```python
from build123d import *

# Parameters (mm, degrees)
F0_W     = 15
F0_H     = 5.5
F0_R     = 2
F0_W_2   = 5.5
F0_H_2   = 15
F0_W_3   = 55
F0_H_3   = 103
F1_DEPTH = 4
F2_R     = 2.5
F3_R     = 5


# Not quite as in the source:
# - a feature names something its author has since deleted; it is built from what else it names


with BuildPart() as f1:
    # F0 (on Top) → F1 (new body)
    with BuildSketch(Plane.XY):
        Polygon((57.5, 63.25), (32.5, 63.25), (-32.5, 63.25), (-32.5, -63.25), (-32.5, -88.25), (57.5, -88.25), align=None)
        with Locations((-12.5, -78.25)):
            Rectangle(F0_W, F0_H, mode=Mode.SUBTRACT)
        with Locations((-26, -56.25)):
            Circle(F0_R, mode=Mode.SUBTRACT)
        with Locations((-0.25, -56.25)):
            Circle(F0_R, mode=Mode.SUBTRACT)
        with Locations((25.5, -56.25)):
            Circle(F0_R, mode=Mode.SUBTRACT)
        with Locations((47.5, -68.25)):
            Rectangle(F0_W_2, F0_H_2, mode=Mode.SUBTRACT)
        Rectangle(F0_W_3, F0_H_3, mode=Mode.SUBTRACT)
        with Locations((-26, 56.75)):
            Circle(F0_R, mode=Mode.SUBTRACT)
        with Locations((-0.25, 56.75)):
            Circle(F0_R, mode=Mode.SUBTRACT)
        with Locations((47.5, -12.5)):
            Rectangle(F0_W_2, F0_H_2, mode=Mode.SUBTRACT)
        with Locations((25.5, 56.75)):
            Circle(F0_R, mode=Mode.SUBTRACT)
        with Locations((47.5, 43.25)):
            Rectangle(F0_W_2, F0_H_2, mode=Mode.SUBTRACT)
    extrude(amount=F1_DEPTH)

    # F2
    f2_edges = [f1.edges().sort_by_distance(p)[0] for p in [
        (-20, -81, 2),
        (-20, -75.5, 2),
        (-5, -75.5, 2),
        (-5, -81, 2),
        (50.25, -60.75, 2),
        (50.25, -75.75, 2),
        (44.75, -75.75, 2),
        (44.75, -60.75, 2),
        (44.75, -5, 2),
        (50.25, -5, 2),
        (50.25, -20, 2),
        (44.75, -20, 2),
        (44.75, 35.75, 2),
        (44.75, 50.75, 2),
        (50.25, 50.75, 2),
        (50.25, 35.75, 2),
    ]]
    fillet(f2_edges, radius=F2_R)

    # F3
    f3_edges = [f1.edges().sort_by_distance(p)[0] for p in [
        (-32.5, 63.25, 2),
        (-32.5, -88.25, 2),
        (57.5, -88.25, 2),
        (57.5, 63.25, 2),
    ]]
    fillet(f3_edges, radius=F3_R)


solid = f1.part
```
Geometry check sheet. Reference: the model listing, model coordinates, mm. A direction names the side the tool comes from. Give positions to 0.01 mm unless a question says otherwise; leave off trailing zeros. Order: outer loops, then holes, each group sorted by start corner. A loop starts at its lowest first (then second) coordinate and runs counter-clockwise, first axis right, second up. Notation, with made-up numbers: (-1.75, 27.5) - (45.25, 27.5) arc R22 cw to (45.25, 63.5) - close; hole circle Ø1 at (3, 18.5). An arc over 180 degrees is marked (long way). Answer in a Markdown table with one row per item. Add a question column.
Q1. Cross-section at C-C, the plane y = 43.5. Enter the section's corners in (x, z).
Q2. Cross-section at A-A, the plane y = 12. Enter the section's corners in (x, z).
Q3. Cross-section at D-D, the plane x = 25.5. Enter the section's corners in (y, z), then the cut area to 3 significant figures.
Q4. Tool access check on faces 4 (the flat face through (44.75, -68, 2)), 5 (the flat face through (57.5, -13, 2)). Record the directions out of +Z, -Z, +X, -X, +Y, -Y that give a thin tool (end or side, any length) a straight path to the whole face; none if there is none.
Q5. Material ranges on probe 1 along Y at (x, z) = (25.5, 1.3); probe 2 along Y at (x, z) = (47, 0.8); probe 3 along X at (y, z) = (-39.5, 3.85), recorded low to high. Write a range as from..to.
Q6. Gauge pin test, flat end, axial feed: pin 1 (2.5 mm diameter, centred on x = 25.5, y = 56.75, fed in from -Z). Record the tip position at first contact, or that the pin passes through.
Q7. Cross-section at B-B, the plane x = -11.5. Enter the section's corners in (y, z).
Q8. Mould release check, pull along Y, two halves, no side actions. Record for faces 1 (the flat face through (44.75, 43, 2)), 2 (the flat face through (32, -11, 4)), 3 (the cylindrical face through (56, 61.82, 2.03)): pulls with the +Y half, pulls with the -Y half, needs draft (parallel to the pull), parting line crosses it, or undercut.
Check values:
| question | item | result |
|---|---|---|
| 1 | outline | (-32.5, 0) - (-27.5, 0) - (-27.5, 4) - (-32.5, 4) - close; (27.5, 0) - (44.75, 0) - (44.75, 4) - (27.5, 4) - close; (50.25, 0) - (57.5, 0) - (57.5, 4) - (50.25, 4) - close |
| 2 | outline | (-32.5, 0) - (-27.5, 0) - (-27.5, 4) - (-32.5, 4) - close; (27.5, 0) - (57.5, 0) - (57.5, 4) - (27.5, 4) - close |
| 3 | outline | (-88.25, 0) - (-58.25, 0) - (-58.25, 4) - (-88.25, 4) - close; (-54.25, 0) - (-51.5, 0) - (-51.5, 4) - (-54.25, 4) - close; (51.5, 0) - (54.75, 0) - (54.75, 4) - (51.5, 4) - close; (58.75, 0) - (63.25, 0) - (63.25, 4) - (58.75, 4) - close |
| 3 | area | 162 mm^2 |
| 4 | face 4 | +Z, -Z |
| 4 | face 5 | +Z, -Z, +X, +Y, -Y |
| 5 | probe 1 | y = -88.25..-58.25, -54.25..-51.5, 51.5..54.75, 58.75..63.25 |
| 5 | probe 2 | y = -88.25..-75.74, -60.76..-19.99, -5.01..35.76, 50.74..63.25 |
| 5 | probe 3 | x = -32.5..-27.5, 27.5..57.5 |
| 6 | pin 1 | passes through |
| 7 | outline | (-88.25, 0) - (-81, 0) - (-81, 4) - (-88.25, 4) - close; (-75.5, 0) - (-51.5, 0) - (-51.5, 4) - (-75.5, 4) - close; (51.5, 0) - (63.25, 0) - (63.25, 4) - (51.5, 4) - close |
| 8 | face 1 | undercut |
| 8 | face 2 | needs draft |
| 8 | face 3 | pulls with the +Y half |
